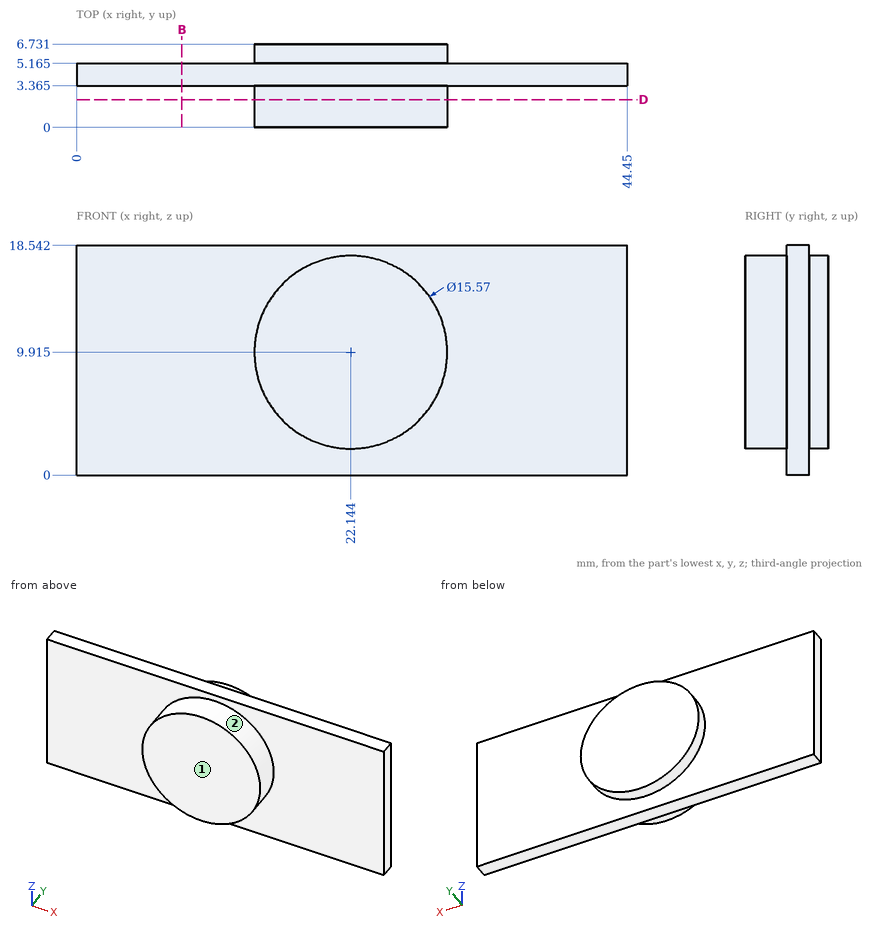
The figure shows three views and two pictorial views of one solid part (mm, origin at its lowest corner). Answer the questions. A direction names the side the tool comes from. Give positions to 0.01 mm unless a question says otherwise; leave off trailing zeros. Order: outer loops, then holes, each group sorted by start corner. A loop starts at its lowest first (then second) coordinate and runs counter-clockwise, first axis right, second up. Notation, with made-up numbers: (61, -11.75) -> (116, -11.75) arc R6 ccw to (116, -2.75) -> close; hole circle Ø10 at (10, 36). An arc over 180 degrees is marked (long way). One line per item, written item: value.
1) Find section D-D, the plane y = 2.25. Determine the outline of the cut face in (x, z) (1 decimal).
Reported:
outline: circle Ø15.6 at (22.1, 9.9)
2) A tool of negligible diameter and unlimited length cuts with its end or side. For the marked faces 1 and 2, from which of +Z, -Z, +X, -X, +Y, -Y can it reach the whole face along a straight path? Write none if from no direction.
Reported:
face 1: +Z, -Z, +X, -X, -Y
face 2: -Y
3) Find the intervals of material crossed by line 1 (Y direction, x = 33.5, z = 8.25) (1 decimal); line 2 (X direction, y = 5.25, z = 8.5); line 3 (X direction, y = 1, z = 15.5) (1 decimal), in increasing order.
Reported:
line 1: y = 3.4 to 5.2
line 2: x = 14.49 to 29.8
line 3: x = 16.7 to 27.6
4) Find section B-B, the plane x = 8.5. Determine the outline of the cut face in (y, z) (1 decimal).
Reported:
outline: (3.4, 0) -> (5.2, 0) -> (5.2, 18.5) -> (3.4, 18.5) -> close
5) Flat-ended cylindrical pins translate along their axes: P1, Ø10, axis at x = 11.5, z = 2.5, coming from the +Y side (1 decimal); P2, Ø3, axis at x = 16, y = 1.5, coming from the -Z side; P3, Ø5, axis at x = 8, z = 16, coming from the -Y side (1 decimal). Find the tip coordinate at first contact, or state that the pin passes through.
Reported:
P1: stops at y = 5.2
P2: stops at z = 3.67
P3: stops at y = 3.4
